```python
from build123d import *

# Parameters (mm, degrees)
F0_W      = 67.939341
F0_H      = 43.90462
F1_DEPTH  = 25
F4_R      = 7.163185
F5_DEPTH  = 5
F2_R      = 7.125778
F6_DEPTH  = 5
F3_R      = 7.157073
F7_DEPTH  = 5
F8_R      = 7.110337
F11_DEPTH = 5
F9_R      = 7.319436
F10_R     = 7.163193
F12_DEPTH = 5


with BuildPart() as f1:
    # F0 (on Top) → F1 (new body)
    with BuildSketch(Plane.XY):
        with Locations((-31.644568, 19.702698)):
            Rectangle(F0_W, F0_H)
    extrude(amount=F1_DEPTH)

    # F4 (on face) → F5 (join)
    with BuildSketch(Plane.XY.offset(25)):
        with Locations((-17.577875, 10.892338)):
            Circle(F4_R)
    extrude(amount=F5_DEPTH)

    # F2 (on face) → F6 (join)
    with BuildSketch(Plane.XY.offset(25)):
        with Locations((-55.946503, 9.800529)):
            Circle(F2_R)
    extrude(amount=F6_DEPTH)

    # F3 (on face) → F7 (join)
    with BuildSketch(Plane.XY.offset(25)):
        with Locations((-37.314776, 9.52596)):
            Circle(F3_R)
    extrude(amount=F7_DEPTH)

    # F8 (on face) → F11 (join)
    with BuildSketch(Plane.XY.offset(25)):
        with Locations((-55.493828, 32.125078)):
            Circle(F8_R)
    extrude(amount=F11_DEPTH)

    # F9 (on face) + F10 (on face) → F12 (join)
    with BuildSketch(Plane.XY.offset(25)):
        with Locations((-36.76331, 29.901806)):
            Circle(F9_R)
    with BuildSketch(Plane.XY.offset(25)):
        with Locations((-15.822439, 30.960426)):
            Circle(F10_R)
    extrude(amount=F12_DEPTH)


solid = f1.part
```
For this review, take the finished solid that the model builds, in its own axes (mm). A direction names the side the tool comes from. Coordinates: 2 decimals unless noted, no trailing zeros. Order: outer loops, then holes, each group sorted by start corner. A loop starts at its lowest first (then second) coordinate and runs counter-clockwise, first axis right, second up. Notation, with made-up numbers: (12.5, -20.5) -> (66.5, -20.5) arc R22 cw to (66.5, 2.5) -> close; hole circle Ø6 at (57.25, -35.5). An arc over 180 degrees is marked (long way). Answer as CSV lines item,"result".
Q1. We need section A-A (x = -41). State the section outline as (y, z) points (3 decimals), plus the area to 3 significant figures.
Model answer:
outline,"(-2.25, 0) -> (41.655, 0) -> (41.655, 25) -> (35.87, 25) -> (35.87, 30) -> (23.933, 30) -> (23.933, 25) -> (15.661, 25) -> (15.661, 30) -> (3.391, 30) -> (3.391, 25) -> (-2.25, 25) -> close"
area,"1,220 mm2"
Q2. Draft analysis for pull direction Y (two halves, no side actions). For faces 3 (the face through (-42.994, 5.171, 27.465)), 4 (the face through (-37, 10, 30)), 5 (the face through (-32, 41.655, 12)), state which applies: released by +Y, released by -Y, zero draft, split by the parting line, or undercut.
Model answer:
face 3,"undercut"
face 4,"zero draft"
face 5,"released by +Y"
Q3. We need section C-C (z = 27.5). State the section outline as (x, y) points.
Model answer:
outline,"circle Ø14.25 at (-55.95, 9.8); circle Ø14.22 at (-55.49, 32.13); circle Ø14.31 at (-37.31, 9.53); circle Ø14.64 at (-36.76, 29.9); circle Ø14.33 at (-17.58, 10.89); circle Ø14.33 at (-15.82, 30.96)"
Q4. We need section D-D (y = 27). State the section outline as (x, z) points.
Model answer:
outline,"(-65.61, 0) -> (2.33, 0) -> (2.33, 25) -> (-9.85, 25) -> (-9.85, 30) -> (-21.79, 30) -> (-21.79, 25) -> (-30.04, 25) -> (-30.04, 30) -> (-43.48, 30) -> (-43.48, 25) -> (-50.57, 25) -> (-50.57, 30) -> (-60.42, 30) -> (-60.42, 25) -> (-65.61, 25) -> close"
Q5. We need section B-B (y = 33). State the section outline as (x, z) points, plus the area to 3 significant figures.
Model answer:
outline,"(-65.61, 0) -> (2.33, 0) -> (2.33, 25) -> (-8.96, 25) -> (-8.96, 30) -> (-22.69, 30) -> (-22.69, 25) -> (-30.13, 25) -> (-30.13, 30) -> (-43.39, 30) -> (-43.39, 25) -> (-48.44, 25) -> (-48.44, 30) -> (-62.55, 30) -> (-62.55, 25) -> (-65.61, 25) -> close"
area,"1,900 mm2"
Q6. Wall thickness on line 1 along Z through (x, y) = (-5, 1.5); line 2 along X through (y, z) = (8, 28.75); line 3 along X through (y, z) = (33.5, 26): over which ranges is each line inside the solid? List them lowest first. Write a range as [from, to].
Model answer:
line 1,"z = [0, 25]"
line 2,"x = [-62.84, -49.05], [-44.31, -30.32], [-24.13, -11.02]"
line 3,"x = [-62.47, -48.52], [-43.14, -30.39], [-22.52, -9.12]"
Q7. For faces 1 (the face through (-10.96, 8.15, 27.46)), 2 (the face through (-65.614, 19, 12)), list the 3-axis set-ups (+Z, -Z, +X, -X, +Y, -Y) from which the entire face can be reached by the end or side of a thin tool; tool diameter is ignored.
Model answer:
face 1,"+Z"
face 2,"+Z, -Z, -X, +Y, -Y"
Q8. Clearance check with a flat-ended pin moving along its axis: pin 1 Ø4 at (x, y) = (-34, 16) entering from +Z. State where the tip first meets the part, or that it passes through.
Model answer:
pin 1,"stops at z = 30"
